Source: CAD feature listing. Evaluate the final solid. Frame: model axes, mm. Face numbers are marked on the shaded views. Give positions to 0.01 mm unless a question says otherwise; leave off trailing zeros. Order: outer loops, then holes, each group sorted by start corner. A loop starts at its lowest first (then second) coordinate and runs counter-clockwise, first axis right, second up. Notation, with made-up numbers: M 28.5,82 L 55.5,82 A25 ccw 55.5,110 Z; hole C 56.25,33.25 d5. An arc over 180 degrees is marked long. Answer as a JSON object with one key per item and string values. Group by question number.
1. Section query A-A (x = 0). Output: boundary loops of the cut face in (y, z).
2. Material intervals for L1, parallel to X at y = 2.65, z = 0; L2, parallel to X at y = 4.65, z = 0; L3, parallel to Z at x = -2, y = 1.45, sorted ascending. Write a range as [from, to].
3. Pull-direction query (X, two-part tool) for the marked faces 1, 2 and 3; classes: +X half, -X half, draft (parallel to the pull), parting line (faces both ways), or undercut.
4. Pin query (flat end, axial travel): P1, Ø2, axis at y = 2.5, z = -4.5, coming from the -X side; P2, Ø1, axis at x = -3.5, y = 1.5, coming from the +Z side; P3, Ø1.5, axis at y = 3, z = -1.5, coming from the +X side. Return the tip coordinate at first contact, or that it passes through.
5. Section query C-C (y = 2). Output: boundary loops of the cut face in (x, z).
6. Section query B-B (z = 7.25). Output: boundary loops of the cut face in (x, y), plus the area to 3 significant figures.
from build123d import *

# Parameters (mm, degrees)
SKETCH1_R               = 9.35
BOSS_EXTRUDE1_DEPTH     = 4.8
CUT_EXTRUDE1_DEPTH      = 15.067160339
CUT_EXTRUDE1_DEPTH_BACK = 15.067160339
SKETCH2_R               = 8.1
SKETCH3_R               = 9
CUT_EXTRUDE2_DEPTH      = 0.3


with BuildPart() as part:
    # Sketch1 → Boss-Extrude1 (new body)
    with BuildSketch(Plane(origin=(0, 0, 0), x_dir=(1, 0, 0), z_dir=(0, 1, 0))):
        with Locations(Location((0, 0, 0), (0, 0, 270))):
            Circle(SKETCH1_R)
    extrude(amount=BOSS_EXTRUDE1_DEPTH)

    # Sketch2 → Cut-Extrude1 (cut, two sides: drawn at the far end of the back side and taken through both)
    with BuildSketch(Plane(origin=(0, 4.8, 0), x_dir=(1, 0, 0), z_dir=(0, 1, 0)).offset(-CUT_EXTRUDE1_DEPTH_BACK)):
        with Locations(Location((0, 0, 0), (0, 0, 270))):
            Circle(SKETCH2_R)
    extrude(amount=CUT_EXTRUDE1_DEPTH + CUT_EXTRUDE1_DEPTH_BACK, mode=Mode.SUBTRACT)

    # Sketch3 → Cut-Extrude2 (cut)
    with BuildSketch(Plane(origin=(0, 4.8, 0), x_dir=(1, 0, 0), z_dir=(0, 1, 0))):
        with Locations(Location((0, 0, 0), (0, 0, 270))):
            Circle(SKETCH3_R)
    extrude(amount=-CUT_EXTRUDE2_DEPTH, mode=Mode.SUBTRACT)


solid = part.part
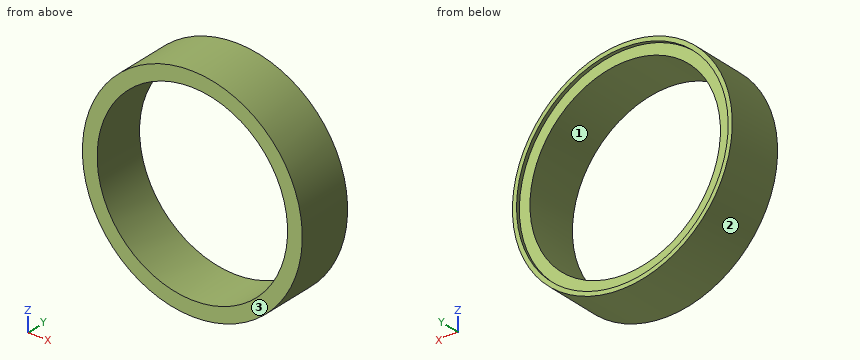
Answer sheet:
{
 "1": {"outline": "M 0,-9.35 L 4.8,-9.35 L 4.8,-9 L 4.5,-9 L 4.5,-8.1 L 0,-8.1 Z; M 0,8.1 L 4.5,8.1 L 4.5,9 L 4.8,9 L 4.8,9.35 L 0,9.35 Z"},
 "2": {"L1": "[-9.35, -8.1], [8.1, 9.35]", "L2": "[-9.35, -9], [9, 9.35]", "L3": "[-9.13, -7.85], [7.85, 9.13]"},
 "3": {"face 1": "undercut", "face 2": "parting line", "face 3": "draft"},
 "4": {"P1": "x = -8.67", "P2": "z = 8.86", "P3": "x = 9.32"},
 "5": {"outline": "C 0,0 d18.7; hole C 0,0 d16.2"},
 "6": {"outline": "M -5.9,0 L -3.61,0 L -3.61,4.5 L -5.33,4.5 L -5.33,4.8 L -5.9,4.8 Z; M 3.61,0 L 5.9,0 L 5.9,4.8 L 5.33,4.8 L 5.33,4.5 L 3.61,4.5 Z", "area": "21.0 mm^2"}
}
